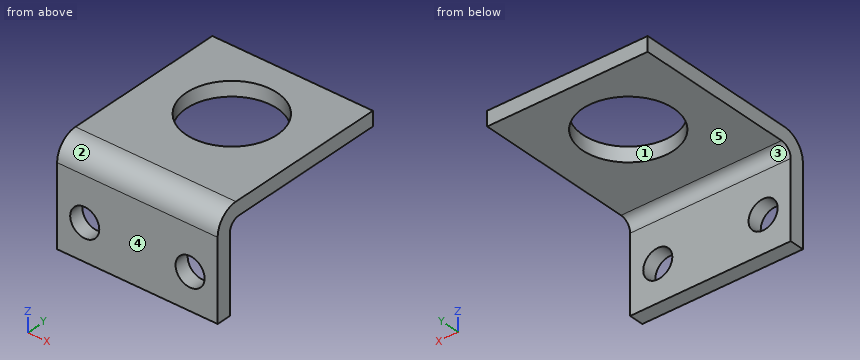
```python
from build123d import *

# Parameters (mm, degrees)
BOSS_EXTRU_1_DEPTH      = 22.1
ESQUISSE2_R             = 2
ENL_V_MAT_EXTRU_1_DEPTH = 3
ESQUISSE3_R             = 6.25
ENL_V_MAT_EXTRU_2_DEPTH = 3


with BuildPart() as part:
    # Esquisse1 → Boss.-Extru.1 (new body)
    with BuildSketch(Plane(origin=(0, 0, 0), x_dir=(0, 0, -1), z_dir=(1, 0, 0))):
        with BuildLine():
            Line((0, 25.5), (0, 3))
            ThreePointArc((0, 3), (0.878679656, 0.878679656), (3, 0))
            Line((3, 0), (14, 0))
            Line((14, 0), (14, 2))
            Line((14, 2), (3.5, 2))
            ThreePointArc((3.5, 2), (2.439339828, 2.439339828), (2, 3.5))
            Line((2, 3.5), (2, 25.5))
            Line((2, 25.5), (0, 25.5))
        make_face()
    extrude(amount=BOSS_EXTRU_1_DEPTH)

    # Esquisse2 → Enlèv. mat.-Extru.1 (cut, through all)
    with BuildSketch(Plane(origin=(0, 2, 0), x_dir=(1, 0, 0), z_dir=(0, 1, 0))):
        with Locations((3.8, 9)):
            Circle(ESQUISSE2_R)
        with Locations((18.3, 9)):
            Circle(ESQUISSE2_R)
    extrude(amount=-ENL_V_MAT_EXTRU_1_DEPTH, mode=Mode.SUBTRACT)

    # Esquisse3 → Enlèv. mat.-Extru.2 (cut, through all)
    with BuildSketch(Plane(origin=(0, 0, -2), x_dir=(-1, 0, 0), z_dir=(0, 0, -1))):
        with Locations((-11.05, 15.5)):
            Circle(ESQUISSE3_R)
    extrude(amount=-ENL_V_MAT_EXTRU_2_DEPTH, mode=Mode.SUBTRACT)


solid = part.part
```
Work out the finished part from the listing and answer in its coordinate system (mm). Face numbers are marked on the shaded views. A direction names the side the tool comes from. Round coordinates to 2 decimals unless told otherwise and drop trailing zeros. Order: outer loops, then holes, each group sorted by start corner. A loop starts at its lowest first (then second) coordinate and runs counter-clockwise, first axis right, second up.
Q1. Find the intervals of material crossed by line 1 along X through (y, z) = (1.1, -9); line 2 along Y through (x, z) = (21, -4.5); line 3 along Y through (x, z) = (9, -1.5), in increasing order.
Solution:
line 1: x = 0 to 1.8, 5.8 to 16.3, 20.3 to 22.1
line 2: y = 0 to 2
line 3: y = 0.4 to 9.6, 21.4 to 25.5
Q2. A tool of negligible diameter and unlimited length cuts with its end or side. For the marked faces 4 and 5, from which of +Z, -Z, +X, -X, +Y, -Y can it reach the whole face along a straight path? Write none if from no direction.
Solution:
face 4: +Z, -Z, +X, -X, -Y
face 5: -Z, +X, -X, +Y
Q3. A cutting plane is placed at D-D, the plane x = 11.05. Determine the outline of the cut face in (y, z), then the cut area to 3 significant figures.
Solution:
outline: (0, -14) - (2, -14) - (2, -3.5) arc R1.5 cw to (3.5, -2) - (9.25, -2) - (9.25, 0) - (3, 0) arc R3 ccw to (0, -3) - close; (21.75, -2) - (25.5, -2) - (25.5, 0) - (21.75, 0) - close
area: 48.6 mm2
Q4. A cutting plane is placed at C-C, the plane z = -9. Determine the outline of the cut face in (x, y).
Solution:
outline: (0, 0) - (1.8, 0) - (1.8, 2) - (0, 2) - close; (5.8, 0) - (16.3, 0) - (16.3, 2) - (5.8, 2) - close; (20.3, 0) - (22.1, 0) - (22.1, 2) - (20.3, 2) - close
Q5. A cutting plane is placed at B-B, the plane y = 15.5. Determine the outline of the cut face in (x, z).
Solution:
outline: (0, -2) - (4.8, -2) - (4.8, 0) - (0, 0) - close; (17.3, -2) - (22.1, -2) - (22.1, 0) - (17.3, 0) - close
Q6. Given pin 1 Ø4 at (x, y) = (18, 6) entering from -Z; pin 2 Ø3.5 at (x, z) = (18.3, -9) entering from +Y, each flat-ended and moving along its own axis, determine where each tip first touches the part or whether it passes through.
Solution:
pin 1: stops at z = -2
pin 2: passes through
Q7. A cutting plane is placed at A-A, the plane x = 3.8. Determine the outline of the cut face in (y, z), then the cut area to 3 significant figures.
Solution:
outline: (0, -14) - (2, -14) - (2, -11) - (0, -11) - close; (0, -7) - (2, -7) - (2, -3.5) arc R1.5 cw to (3.5, -2) - (25.5, -2) - (25.5, 0) - (3, 0) arc R3 ccw to (0, -3) - close
area: 65.6 mm2
Q8. The mould has two halves that part along Y. Classify the marked faces 1, 2 and 3: pulls with the +Y half, pulls with the -Y half, needs draft (parallel to the pull), parting line crosses it, or undercut.
Solution:
face 1: undercut
face 2: pulls with the -Y half
face 3: pulls with the +Y half
